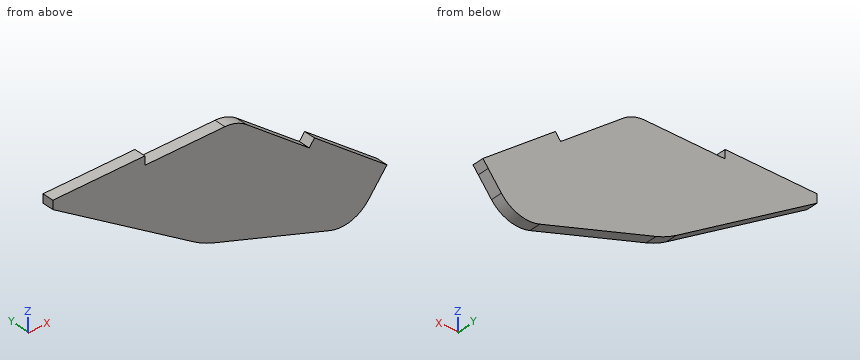
from build123d import *

# Parameters (mm, degrees)
BOSS_EXTRUDE1_DEPTH = 3.175
SKETCH2_W           = 25.4
SKETCH2_H           = 2.38125
BOSS_EXTRUDE2_DEPTH = 3.175
FILLET1_R           = 9.525
CUT_EXTRUDE1_DEPTH  = 4.175
FILLET2_R           = 25.4


with BuildPart() as part:
    # Sketch1 → Boss-Extrude1 (new body)
    with BuildSketch(Plane(origin=(0, 0, 0), x_dir=(1, 0, 0), z_dir=(0, 1, 0))):
        Polygon((-50.8, 0), (0, 0), (40.030946283, 31.275602947), (32.212045547, 41.283339517), (-50.8, 12.7), align=None)
    extrude(amount=BOSS_EXTRUDE1_DEPTH)

    # Sketch2 → Boss-Extrude2 (add)
    with BuildSketch(Plane(origin=(0, 3.175, 0), x_dir=(1, 0, 0), z_dir=(0, 1, 0))):
        Polygon((20.015473142, 15.637801473), (40.030946283, 31.275602947), (41.496990171, 29.39915234), (21.48151703, 13.761350866), align=None)
        with Locations((-38.1, -1.190625)):
            Rectangle(SKETCH2_W, SKETCH2_H)
    extrude(amount=-BOSS_EXTRUDE2_DEPTH)

    # Fillet1
    fillet1_edges = [part.edges().sort_by_distance(p)[0] for p in [
        (-50.8, 1.5875, -12.7),
        (32.212045547, 1.5875, -41.283339517),
        (0, 1.5875, 0),
    ]]
    fillet(fillet1_edges, radius=FILLET1_R)

    # Sketch3 → Cut-Extrude1 (cut, through all)
    with BuildSketch(Plane(origin=(0, 3.175, 0), x_dir=(1, 0, 0), z_dir=(0, 1, 0))):
        with BuildLine():
            Line((-50.8, 0), (-9.293977227, 26.991669759))
            Line((-9.293977227, 26.991669759), (-44.376036671, 14.911947961))
            ThreePointArc((-44.376036671, 14.911947961), (-49.029450312, 11.437079181), (-50.8, 5.905883528))
            Line((-50.8, 5.905883528), (-50.8, 0))
        make_face()
    extrude(amount=-CUT_EXTRUDE1_DEPTH, mode=Mode.SUBTRACT)

    # Fillet2
    fillet2_edges = [part.edges().sort_by_distance(p)[0] for p in [
        (-9.293977227, 1.5875, -26.991669759),
    ]]
    fillet(fillet2_edges, radius=FILLET2_R)


solid = part.part
The listing builds one solid part. Answer for the finished solid, in the listing's coordinates (mm). Round coordinates to 2 decimals unless told otherwise and drop trailing zeros. Order: outer loops, then holes, each group sorted by start corner. A loop starts at its lowest first (then second) coordinate and runs counter-clockwise, first axis right, second up. Notation, with made-up numbers: M 33,17.25 L 52,17.25 A22 cw 52,43.25 Z; hole C -30.75,4 d1. An arc over 180 degrees is marked long. Answer in a Markdown table with one row per item. Add a question column.
1) Flat-ended cylindrical pins translate along their axes: pin 1 Ø1 at (x, y) = (-13, 1) entering from +Z; pin 2 Ø1.5 at (y, z) = (1, -29) entering from +X; pin 3 Ø1.5 at (x, y) = (-8, 2) entering from -Z. Find the tip coordinate at first contact, or state that the pin passes through.
2) Consider line 1 along Z through (x, y) = (14, 0.3); line 2 along X through (y, z) = (2.7, -8); line 3 along Z through (x, y) = (15, 1.7). Determine where each line is inside the solid, lowest interval first. Write a range as from..to.
3) The part is cut by section B-B on z = -16.5. Determine the outline of the cut face in (x, y) (3 decimals).
4) The part is cut by section C-C on x = -1.5. Determine the outline of the cut face in (y, z) (3 decimals).
Findings below:
| question | item | result |
|---|---|---|
| 1 | pin 1 | stops at z = 0 |
| 1 | pin 2 | stops at x = 41.5 |
| 1 | pin 3 | stops at z = -27.68 |
| 2 | line 1 | z = -35.01..-10.94 |
| 2 | line 2 | x = -38.5..10.24 |
| 2 | line 3 | z = -35.36..-11.72 |
| 3 | outline | M -25.427,0 L 24.987,0 L 24.987,3.175 L -25.427,3.175 Z |
| 4 | outline | M 0,-29.675 L 3.175,-29.675 L 3.175,-0.168 L 0,-0.168 Z |
